```python
from build123d import *

# Parameters (mm, degrees)
CYLINDER076_R           = 13
CYLINDER076_DEPTH       = 2.2
CYLINDER076_ROLL_ANGLE  = 90
CYLINDER075_W           = 14
CYLINDER075_H           = 2
CYLINDER075_ANGLE       = 180
CYLINDER075_ROLL_ANGLE  = 90
CYLINDER029_R           = 6
CYLINDER029_DEPTH       = 20
CYLINDER029_PITCH_ANGLE = 90
CYLINDER030_R           = 6
CYLINDER030_DEPTH       = 20
CYLINDER030_PITCH_ANGLE = 90
CYLINDER028_R           = 13
CYLINDER028_DEPTH       = 50
CYLINDER028_ROLL_ANGLE  = 90
CYLINDER027_R           = 8
CYLINDER027_DEPTH       = 3
CYLINDER027_PITCH_ANGLE = 90
CYLINDER026_R           = 6
CYLINDER026_DEPTH       = 39
CYLINDER026_PITCH_ANGLE = 90
CYLINDER025_R           = 8.25
CYLINDER025_DEPTH       = 33
CYLINDER025_PITCH_ANGLE = 90
CYLINDER024_R           = 11.25
CYLINDER024_DEPTH       = 36
CYLINDER024_PITCH_ANGLE = 90
BOX009_W                = 10
BOX009_H                = 6
BOX009_DEPTH            = 2.7
CYLINDER023_R           = 3
CYLINDER023_DEPTH       = 11
CYLINDER022_R           = 2
CYLINDER022_DEPTH       = 29
BOX008_W                = 10
BOX008_H                = 6
BOX008_DEPTH            = 2.7
CYLINDER021_R           = 3
CYLINDER021_DEPTH       = 11
CYLINDER020_R           = 2
CYLINDER020_DEPTH       = 22
BOX017_W                = 15
BOX017_H                = 6
BOX017_DEPTH            = 3
CYLINDER056_R           = 1.5
CYLINDER056_DEPTH       = 25
CYLINDER055_R           = 2
CYLINDER055_DEPTH       = 32
CYLINDER046_R           = 5
CYLINDER046_DEPTH       = 2.2
CYLINDER046_ROLL_ANGLE  = 90
BOX005_W                = 15
BOX005_H                = 18
BOX005_DEPTH            = 15
BOX005_PITCH_ANGLE      = 45
CYLINDER015_R           = 6
CYLINDER015_DEPTH       = 32
CYLINDER015_ROLL_ANGLE  = 90
BOX004_W                = 6
BOX004_H                = 32
BOX004_DEPTH            = 6
BOX003_W                = 19
BOX003_H                = 32
BOX003_DEPTH            = 3.5
BOX001_W                = 42
BOX001_H                = 42
BOX001_DEPTH            = 16
CYLINDER047_R           = 4
CYLINDER047_DEPTH       = 8


with BuildPart() as obj1:
    # Cylinder076 → Cylinder076 (new body)
    with BuildSketch(Plane.XY):
        Circle(CYLINDER076_R)
    extrude(amount=CYLINDER076_DEPTH)


with BuildPart() as obj1_1:
    # Cylinder076 roll: moved
    add(obj1.part.rotate(Axis((0, 0, 0), (1, 0, 0)), CYLINDER076_ROLL_ANGLE))


with BuildPart() as obj1_2:
    # Cylinder076 placement: moved
    add(obj1_1.part.moved(Location((15, 29, 0))))


with BuildPart() as obj2:
    # Cylinder075 → Cylinder075 (revolve)
    with BuildSketch(Plane.XZ):
        with Locations((7, 1)):
            Rectangle(CYLINDER075_W, CYLINDER075_H)
    revolve(axis=Axis((0, 0, 0), (0, 0, 1)), revolution_arc=CYLINDER075_ANGLE)


with BuildPart() as obj2_1:
    # Cylinder075 roll: moved
    add(obj2.part.rotate(Axis((0, 0, 0), (1, 0, 0)), CYLINDER075_ROLL_ANGLE))


with BuildPart() as obj2_2:
    # Cylinder075 placement: moved
    add(obj2_1.part.moved(Location((15, 29, 0))))

    # Cut010005: cut obj1
    add(obj1_2.part, mode=Mode.SUBTRACT)


with BuildPart() as obj2_3:
    # Cut010005 placement: moved
    add(obj2_2.part.moved(Location((0, -1, 0))))


with BuildPart() as cylinder029:
    # Cylinder029 → Cylinder029 (new body)
    with BuildSketch(Plane.XY):
        Circle(CYLINDER029_R)
    extrude(amount=CYLINDER029_DEPTH)


with BuildPart() as cylinder029_1:
    # Cylinder029 pitch: moved
    add(cylinder029.part.rotate(Axis((0, 0, 0), (0, 1, 0)), CYLINDER029_PITCH_ANGLE))


with BuildPart() as cylinder029_2:
    # Cylinder029 placement: moved
    add(cylinder029_1.part.moved(Location((5, 0, 17.7))))


with BuildPart() as fusion019:
    # Cylinder030 → Cylinder030 (new body)
    with BuildSketch(Plane.XY):
        Circle(CYLINDER030_R)
    extrude(amount=CYLINDER030_DEPTH)


with BuildPart() as fusion019_1:
    # Cylinder030 pitch: moved
    add(fusion019.part.rotate(Axis((0, 0, 0), (0, 1, 0)), CYLINDER030_PITCH_ANGLE))


with BuildPart() as fusion019_2:
    # Cylinder030 placement: moved
    add(fusion019_1.part.moved(Location((5, 0, -17.7))))

    # Fusion019: union Cylinder029
    add(cylinder029_2.part)


with BuildPart() as cut003:
    # Cylinder028 → Cylinder028 (new body)
    with BuildSketch(Plane.XY):
        Circle(CYLINDER028_R)
    extrude(amount=CYLINDER028_DEPTH)


with BuildPart() as cut003_1:
    # Cylinder028 roll: moved
    add(cut003.part.rotate(Axis((0, 0, 0), (1, 0, 0)), CYLINDER028_ROLL_ANGLE))


with BuildPart() as cut003_2:
    # Cylinder028 placement: moved
    add(cut003_1.part.moved(Location((15, 29, 0))))

    # Cut003: cut Fusion019
    add(fusion019_2.part, mode=Mode.SUBTRACT)


with BuildPart() as cylinder027:
    # Cylinder027 → Cylinder027 (new body)
    with BuildSketch(Plane.XY):
        Circle(CYLINDER027_R)
    extrude(amount=CYLINDER027_DEPTH)


with BuildPart() as cylinder027_1:
    # Cylinder027 pitch: moved
    add(cylinder027.part.rotate(Axis((0, 0, 0), (0, 1, 0)), CYLINDER027_PITCH_ANGLE))


with BuildPart() as cylinder027_2:
    # Cylinder027 placement: moved
    add(cylinder027_1.part.moved(Location((39, 0, 0))))


with BuildPart() as cylinder026:
    # Cylinder026 → Cylinder026 (new body)
    with BuildSketch(Plane.XY):
        Circle(CYLINDER026_R)
    extrude(amount=CYLINDER026_DEPTH)


with BuildPart() as cylinder026_1:
    # Cylinder026 pitch: moved
    add(cylinder026.part.rotate(Axis((0, 0, 0), (0, 1, 0)), CYLINDER026_PITCH_ANGLE))


with BuildPart() as cylinder026_2:
    # Cylinder026 placement: moved
    add(cylinder026_1.part)


with BuildPart() as cylinder025:
    # Cylinder025 → Cylinder025 (new body)
    with BuildSketch(Plane.XY):
        Circle(CYLINDER025_R)
    extrude(amount=CYLINDER025_DEPTH)


with BuildPart() as cylinder025_1:
    # Cylinder025 pitch: moved
    add(cylinder025.part.rotate(Axis((0, 0, 0), (0, 1, 0)), CYLINDER025_PITCH_ANGLE))


with BuildPart() as cylinder025_2:
    # Cylinder025 placement: moved
    add(cylinder025_1.part)


with BuildPart() as obj3:
    # Cylinder024 → Cylinder024 (new body)
    with BuildSketch(Plane.XY):
        Circle(CYLINDER024_R)
    extrude(amount=CYLINDER024_DEPTH)


with BuildPart() as obj3_1:
    # Cylinder024 pitch: moved
    add(obj3.part.rotate(Axis((0, 0, 0), (0, 1, 0)), CYLINDER024_PITCH_ANGLE))


with BuildPart() as obj3_2:
    # Cylinder024 placement: moved
    add(obj3_1.part.moved(Location((-6, 0, 0))))

    # Fusion020: union Cut003, Cylinder027, Cylinder026, Cylinder025
    add(cut003_2.part)
    add(cylinder027_2.part)
    add(cylinder026_2.part)
    add(cylinder025_2.part)


with BuildPart() as cube006:
    # Box009 → Box009 (new body)
    with BuildSketch(Plane(origin=(41.8, 14, -7.5), x_dir=(1, 0, 0), z_dir=(0, 0, 1))):
        with Locations((5, 3)):
            Rectangle(BOX009_W, BOX009_H)
    extrude(amount=BOX009_DEPTH)


with BuildPart() as cylinder023:
    # Cylinder023 → Cylinder023 (new body)
    with BuildSketch(Plane(origin=(45, 21, -6), x_dir=(1, 0, 0), z_dir=(0, 0, 1))):
        Circle(CYLINDER023_R)
    extrude(amount=CYLINDER023_DEPTH)


with BuildPart() as fusion017:
    # Cylinder022 → Cylinder022 (new body)
    with BuildSketch(Plane(origin=(45, 21, -34), x_dir=(1, 0, 0), z_dir=(0, 0, 1))):
        Circle(CYLINDER022_R)
    extrude(amount=CYLINDER022_DEPTH)

    # Fusion016: union Cylinder023
    add(cylinder023.part)


with BuildPart() as fusion017_1:
    # Fusion016 placement: moved
    add(fusion017.part.moved(Location((0, -4, 24))))

    # Fusion017: union Cube006
    add(cube006.part)


with BuildPart() as fusion017_2:
    # Fusion017 placement: moved
    add(fusion017_1.part.moved(Location((-9, -29, 0))))


with BuildPart() as cube005:
    # Box008 → Box008 (new body)
    with BuildSketch(Plane(origin=(41.8, 14, -7.5), x_dir=(1, 0, 0), z_dir=(0, 0, 1))):
        with Locations((5, 3)):
            Rectangle(BOX008_W, BOX008_H)
    extrude(amount=BOX008_DEPTH)


with BuildPart() as cylinder021:
    # Cylinder021 → Cylinder021 (new body)
    with BuildSketch(Plane(origin=(45, 21, -12), x_dir=(1, 0, 0), z_dir=(0, 0, 1))):
        Circle(CYLINDER021_R)
    extrude(amount=CYLINDER021_DEPTH)


with BuildPart() as obj4:
    # Cylinder020 → Cylinder020 (new body)
    with BuildSketch(Plane(origin=(45, 21, -34), x_dir=(1, 0, 0), z_dir=(0, 0, 1))):
        Circle(CYLINDER020_R)
    extrude(amount=CYLINDER020_DEPTH)

    # Fusion014: union Cylinder021
    add(cylinder021.part)


with BuildPart() as obj4_1:
    # Fusion014 placement: moved
    add(obj4.part.moved(Location((0, -4, 24))))

    # Fusion015: union Cube005
    add(cube005.part)


with BuildPart() as obj4_2:
    # Fusion015 placement: moved
    add(obj4_1.part.moved(Location((-9, 3, 0))))

    # Fusion018: union Fusion017
    add(fusion017_2.part)


with BuildPart() as cube014:
    # Box017 → Box017 (new body)
    with BuildSketch(Plane(origin=(58.2, 67, 3), x_dir=(1, 0, 0), z_dir=(0, 0, 1))):
        with Locations((7.5, 3)):
            Rectangle(BOX017_W, BOX017_H)
    extrude(amount=BOX017_DEPTH)


with BuildPart() as cylinder056:
    # Cylinder056 → Cylinder056 (new body)
    with BuildSketch(Plane(origin=(70, 70, 7), x_dir=(1, 0, 0), z_dir=(0, 0, 1))):
        Circle(CYLINDER056_R)
    extrude(amount=CYLINDER056_DEPTH)


with BuildPart() as obj5:
    # Cylinder055 → Cylinder055 (new body)
    with BuildSketch(Plane(origin=(70, 70, 0), x_dir=(1, 0, 0), z_dir=(0, 0, 1))):
        Circle(CYLINDER055_R)
    extrude(amount=CYLINDER055_DEPTH)

    # Fusion040: union Cube014, Cylinder056
    add(cube014.part)
    add(cylinder056.part)


with BuildPart() as obj5_1:
    # Fusion040 placement: moved
    add(obj5.part.moved(Location((-70, -48, 7))))


with BuildPart() as obj6:
    # Cylinder046 → Cylinder046 (new body)
    with BuildSketch(Plane.XY):
        Circle(CYLINDER046_R)
    extrude(amount=CYLINDER046_DEPTH)


with BuildPart() as obj6_1:
    # Cylinder046 roll: moved
    add(obj6.part.rotate(Axis((0, 0, 0), (1, 0, 0)), CYLINDER046_ROLL_ANGLE))


with BuildPart() as obj6_2:
    # Cylinder046 placement: moved
    add(obj6_1.part.moved(Location((15, 26, 0))))

    # Fusion052: union obj3, obj4, obj5
    add(obj3_2.part)
    add(obj4_2.part)
    add(obj5_1.part)


with BuildPart() as cube002:
    # Box005 → Box005 (new body)
    with BuildSketch(Plane.XY):
        with Locations((7.5, 9)):
            Rectangle(BOX005_W, BOX005_H)
    extrude(amount=BOX005_DEPTH)


with BuildPart() as cube002_1:
    # Box005 pitch: moved
    add(cube002.part.rotate(Axis((0, 0, 0), (0, 1, 0)), BOX005_PITCH_ANGLE))


with BuildPart() as cube002_2:
    # Box005 placement: moved
    add(cube002_1.part.moved(Location((-30, -9, 17))))


with BuildPart() as cylinder015:
    # Cylinder015 → Cylinder015 (new body)
    with BuildSketch(Plane.XY):
        Circle(CYLINDER015_R)
    extrude(amount=CYLINDER015_DEPTH)


with BuildPart() as cylinder015_1:
    # Cylinder015 roll: moved
    add(cylinder015.part.rotate(Axis((0, 0, 0), (1, 0, 0)), CYLINDER015_ROLL_ANGLE))


with BuildPart() as cylinder015_2:
    # Cylinder015 placement: moved
    add(cylinder015_1.part.moved(Location((-6, 16, 6.5))))


with BuildPart() as cut001:
    # Box004 → Box004 (new body)
    with BuildSketch(Plane(origin=(-6, -16, 6.5), x_dir=(1, 0, 0), z_dir=(0, 0, 1))):
        with Locations((3, 16)):
            Rectangle(BOX004_W, BOX004_H)
    extrude(amount=BOX004_DEPTH)

    # Cut001: cut Cylinder015
    add(cylinder015_2.part, mode=Mode.SUBTRACT)


with BuildPart() as cut002:
    # Box003 → Box003 (new body)
    with BuildSketch(Plane(origin=(-19, -16, 12.5), x_dir=(1, 0, 0), z_dir=(0, 0, 1))):
        with Locations((9.5, 16)):
            Rectangle(BOX003_W, BOX003_H)
    extrude(amount=BOX003_DEPTH)

    # Fusion007: union Cut001
    add(cut001.part)

    # Cut002: cut Cube002
    add(cube002_2.part, mode=Mode.SUBTRACT)


with BuildPart() as fusion008:
    # Box001 → Box001 (new body)
    with BuildSketch(Plane(origin=(0, -16, 0), x_dir=(1, 0, 0), z_dir=(0, 0, 1))):
        with Locations((21, 21)):
            Rectangle(BOX001_W, BOX001_H)
    extrude(amount=BOX001_DEPTH)

    # Fusion008: union Cut002
    add(cut002.part)


with BuildPart() as obj7:
    # Cylinder047 → Cylinder047 (new body)
    with BuildSketch(Plane(origin=(0, 22, 8), x_dir=(1, 0, 0), z_dir=(0, 0, 1))):
        Circle(CYLINDER047_R)
    extrude(amount=CYLINDER047_DEPTH)

    # Fusion049: union Fusion008
    add(fusion008.part)

    # Cut010: cut obj6
    add(obj6_2.part, mode=Mode.SUBTRACT)

    # Fusion058: union obj2
    add(obj2_3.part)


solid = obj7.part
```
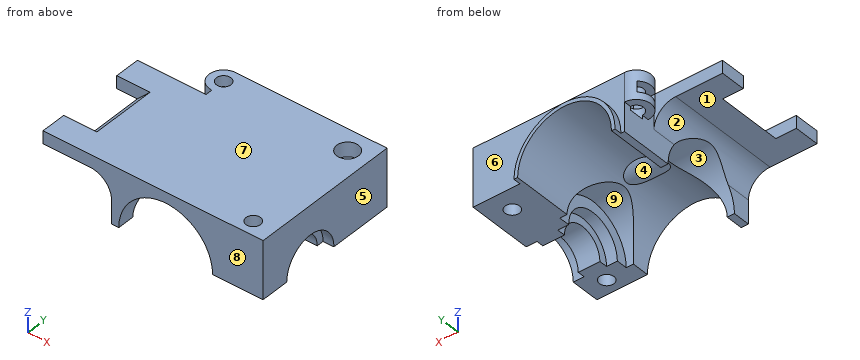
The model under review builds one solid part; all positions refer to its coordinate system, in mm. Face numbers are marked on the shaded views. A direction names the side the tool comes from. Give positions to 0.01 mm unless a question says otherwise; leave off trailing zeros. Write each loop counter-clockwise with the first axis right and the second up, starting at its lowest first coordinate (ties: lowest second). Pieces come first, ordered by that corner, then holes. Notation, with made-up numbers: M 48,-26 L 64,-26 A29 ccw 64,-3 Z; hole C -29,49 d9. An arc over 180 degrees is marked long. Write item = value, one per line. Start each with the question number.
Q1. We need section D-D (y = 0). State the section outline as (x, z) points.
Q2. We need section A-A (x = 15). State the section outline as (y, z) points.
Q3. Machinability: for the marked faces 1, 2, 3, 4 and 5, which of the approach directions +Z, -Z, +X, -X, +Y, -Y give a long, thin tool a straight path to every point of the face, cutting with its end or side? Answer none if there is none.
Q4. Clearance check with flat-ended pins moving along their axes: pin 1 (5 mm diameter, centred on y = -13.5, z = 2, fed in from -X); pin 2 (2.5 mm diameter, centred on y = 0, z = 3, fed in from -X); pin 3 (6.5 mm diameter, centred on x = 35.5, y = 20, fed in from +Z); pin 4 (12 mm diameter, centred on x = 10.5, y = 20, fed in from -Z). State where each tip first meets the part, or that it passes through.
Q5. We need section C-C (z = 2.25). Give the number of separate pieces and of enclosed holes in the cut face, plus the area to 3 significant figures.
Q6. Mouldability with a two-part tool opening along Y and no side actions: class the marked faces 6, 7, 8 and 9 as released by +Y, released by -Y, zero draft, split by the parting line, or undercut.
Q7. For line 1 (Y direction, x = 36, z = 13.8); line 2 (Y direction, x = 35, z = 10.25); line 3 (X direction, y = 22, z = 14.85), list the stretches that pass through material, from the lowest coordinate up.
Q8. We need section B-B (y = 14). State the section outline as (x, z) points.
Result set:
q1.outline = M -13.29,12.5 L -6,12.5 A6 cw -2.33,11.25 L 8.49,11.25 A13 cw 9.33,11.7 L 20.67,11.7 A13 cw 21.51,11.25 L 30,11.25 L 30,8.25 L 33,8.25 L 33,6 L 39,6 L 39,8 L 42,8 L 42,16 L -9.79,16 Z
q2.outline = M -16,13 L -3.73,13 A6 ccw 3.73,13 L 28,13 L 28,14 L 26,14 L 26,16 L -16,16 Z
q3.face_1 = -Z, -X, +Y, -Y
q3.face_2 = -Z, -X, -Y
q3.face_3 = -Z, -X
q3.face_4 = -Z
q3.face_5 = +Z, -Z, +X, +Y, -Y
q4.pin_1 = 0
q4.pin_2 = through
q4.pin_3 = 16
q4.pin_4 = 7.66
q5.separate_pieces = 4
q5.enclosed_holes = 2
q5.area = 410 mm2
q6.face_6 = released by +Y
q6.face_7 = zero draft
q6.face_8 = released by -Y
q6.face_9 = undercut
q7.line_1 = -16 to -14, -10 to 17, 23 to 26
q7.line_2 = -16 to -13.73, -10.27 to 18.27, 21.73 to 26
q7.line_3 = -4 to -2, 2 to 33.76, 38.24 to 42
q8.outline = M -19,12.5 L -6,12.5 A6 cw 0,6.5 L 0,0 L 2,0 A13 cw 28,0 L 42,0 L 42,16 L -19,16 Z
